The model under review builds one solid part; all positions refer to its coordinate system, in mm. Face numbers are marked on the shaded views. A direction names the side the tool comes from. Round coordinates to 2 decimals unless told otherwise and drop trailing zeros. Write each loop counter-clockwise with the first axis right and the second up, starting at its lowest first coordinate (ties: lowest second). Pieces come first, ordered by that corner, then holes. Notation, with made-up numbers: (45.5, -32.5) -> (93.5, -32.5) arc R16 ccw to (93.5, -24.5) -> close; hole circle Ø10 at (57.5, -13). An arc over 180 degrees is marked (long way). Return JSON: item names as keys, results as strings. Group by question number.
1. Take a section at B-B, the plane x = 4.75. Write out the cut boundary in (y, z), then the cut area to 3 significant figures.
2. Tool access review of the marked faces 1 and 2: name each direction out of +Z, -Z, +X, -X, +Y, -Y from which nothing blocks a thin tool from reaching the whole face with its end or side.
3. Clearance check with flat-ended pins moving along their axes: P1, Ø2, axis at y = 178.55, z = -10.5, coming from the -X side; P2, Ø0.6, axis at x = 1, y = 88.5, coming from the -Z side; P3, Ø5.5, axis at x = 11, y = 3.5, coming from the +Z side; P4, Ø5.5, axis at y = 125.12, z = -10.5, coming from the +X side. State where each tip first meets the part, or that it passes through.
4. For line 1 along Y through (x, z) = (1.2, -19); line 2 along X through (y, z) = (195, -1.65); line 3 along Z through (x, y) = (1.5, 151), list the stretches that pass through material, from the lowest coordinate up. Write a range as from..to.
5. Take a section at A-A, the plane y = 58.5. Write out the cut boundary in (x, z).
from build123d import *

# Parameters (mm, degrees)
BOSS_EXTRUDE1_DEPTH                             = 211
CSK_FOR_M3_FLAT_HEAD_MACHINE_SCREW1_D           = 3.4
CSK_FOR_M3_FLAT_HEAD_MACHINE_SCREW1_CSINK_D     = 6.3
CSK_FOR_M3_FLAT_HEAD_MACHINE_SCREW1_CSINK_ANGLE = 90
SKETCH6_W                                       = 7
SKETCH6_H                                       = 10
CUT_EXTRUDE1_DEPTH                              = 213.063669684
SKETCH7_W                                       = 7
SKETCH7_H                                       = 2.5
CUT_EXTRUDE2_DEPTH                              = 213.063669684
CSK_FOR_M3_FLAT_HEAD_MACHINE_SCREW2_D           = 3.4
CSK_FOR_M3_FLAT_HEAD_MACHINE_SCREW2_CSINK_D     = 6.3
CSK_FOR_M3_FLAT_HEAD_MACHINE_SCREW2_CSINK_ANGLE = 90
CSK_FOR_M3_FLAT_HEAD_MACHINE_SCREW3_D           = 3.4
CSK_FOR_M3_FLAT_HEAD_MACHINE_SCREW3_CSINK_D     = 6.3
CSK_FOR_M3_FLAT_HEAD_MACHINE_SCREW3_CSINK_ANGLE = 90
FILLET1_R                                       = 0.5
FILLET2_R                                       = 1
CUT_EXTRUDE3_START                              = -10
SKETCH16_R                                      = 1.7
CUT_EXTRUDE3_DEPTH                              = 10
CUT_EXTRUDE4_START                              = -10
SKETCH17_R                                      = 1.7
CUT_EXTRUDE4_DEPTH                              = 10
SKETCH20_W                                      = 2
SKETCH20_H                                      = 7.5
BOSS_EXTRUDE2_DEPTH                             = 8
SKETCH21_R                                      = 1.7
CUT_EXTRUDE5_DEPTH                              = 3


with BuildPart() as part:
    # Sketch1 → Boss-Extrude1 (new body)
    with BuildSketch(Plane(origin=(0, 0, 0), x_dir=(1, 0, 0), z_dir=(0, 1, 0))):
        Polygon((0, 15), (0, 0), (15, 0), (15, 2), (2, 2), (2, 15), align=None)
    extrude(amount=BOSS_EXTRUDE1_DEPTH)

    # CSK for M3 Flat Head Machine Screw1 (through all)
    with Locations(Plane.ZY):
        with Locations((-10.5, 178.5483), (-10.5, 150.81169946), (-10.5, 125.12070188), (-10.5, 91.71900188), (-10.5, 32.45070188), (-10.5, 79.86070188), (-10.5, 137.8117)):
            CounterSinkHole(CSK_FOR_M3_FLAT_HEAD_MACHINE_SCREW1_D / 2, CSK_FOR_M3_FLAT_HEAD_MACHINE_SCREW1_CSINK_D / 2, counter_sink_angle=CSK_FOR_M3_FLAT_HEAD_MACHINE_SCREW1_CSINK_ANGLE)

    # Sketch6 → Cut-Extrude1 (cut, through all)
    with BuildSketch(Plane.XY):
        with Locations((11.5, 206)):
            Rectangle(SKETCH6_W, SKETCH6_H)
    extrude(amount=-CUT_EXTRUDE1_DEPTH, mode=Mode.SUBTRACT)

    # Sketch7 → Cut-Extrude2 (cut, through all)
    with BuildSketch(Plane.ZY):
        with Locations((-11.5, 202.25)):
            Rectangle(SKETCH7_W, SKETCH7_H)
    extrude(amount=-CUT_EXTRUDE2_DEPTH, mode=Mode.SUBTRACT)

    # CSK for M3 Flat Head Machine Screw2 (through all)
    with Locations(Plane.ZY):
        with Locations((-11, 207.5)):
            CounterSinkHole(CSK_FOR_M3_FLAT_HEAD_MACHINE_SCREW2_D / 2, CSK_FOR_M3_FLAT_HEAD_MACHINE_SCREW2_CSINK_D / 2, counter_sink_angle=CSK_FOR_M3_FLAT_HEAD_MACHINE_SCREW2_CSINK_ANGLE)

    # CSK for M3 Flat Head Machine Screw3 (through all)
    with Locations(Plane.XY):
        with Locations((11, 3.5), (10.5, 195)):
            CounterSinkHole(CSK_FOR_M3_FLAT_HEAD_MACHINE_SCREW3_D / 2, CSK_FOR_M3_FLAT_HEAD_MACHINE_SCREW3_CSINK_D / 2, counter_sink_angle=CSK_FOR_M3_FLAT_HEAD_MACHINE_SCREW3_CSINK_ANGLE)

    # Fillet1
    fillet1_edges = [part.edges().sort_by_distance(p)[0] for p in [
        (0, 105.5, 0),
    ]]
    fillet(fillet1_edges, radius=FILLET1_R)

    # Fillet2
    fillet2_edges = [part.edges().sort_by_distance(p)[0] for p in [
        (2, 105.5, -2),
        (8, 201, -1),
        (1, 203.5, -8),
        (1, 201, -8),
    ]]
    fillet(fillet2_edges, radius=FILLET2_R)

    # Sketch16 → Cut-Extrude3 (cut)
    with BuildSketch(Plane.ZY.offset(CUT_EXTRUDE3_START)):
        with Locations((-10.5, 186.68)):
            Circle(SKETCH16_R)
        with Locations((-10.5, 111.59)):
            Circle(SKETCH16_R)
        with Locations((-10.5, 3)):
            Circle(SKETCH16_R)
        with Locations((-10.5, 178.5483)):
            Circle(SKETCH16_R)
    extrude(amount=CUT_EXTRUDE3_DEPTH, mode=Mode.SUBTRACT)

    # Sketch17 → Cut-Extrude4 (cut)
    with BuildSketch(Plane.XY.offset(CUT_EXTRUDE4_START)):
        with Locations((10.5, 186.68)):
            Circle(SKETCH17_R)
        with Locations((10.5, 111.59)):
            Circle(SKETCH17_R)
        with Locations((10.5, 10)):
            Circle(SKETCH17_R)
        with Locations((10.5, 195)):
            Circle(SKETCH17_R)
    extrude(amount=CUT_EXTRUDE4_DEPTH, mode=Mode.SUBTRACT)

    # Sketch20 → Boss-Extrude2 (add)
    with BuildSketch(Plane(origin=(0, 0, -15), x_dir=(-1, 0, 0), z_dir=(0, 0, -1))):
        with Locations((-1, 207.25)):
            Rectangle(SKETCH20_W, SKETCH20_H)
    extrude(amount=BOSS_EXTRUDE2_DEPTH)

    # Sketch21 → Cut-Extrude5 (cut)
    with BuildSketch(Plane(origin=(2, 0, 0), x_dir=(0, 0, -1), z_dir=(1, 0, 0))):
        with Locations((19, 207.5)):
            Circle(SKETCH21_R)
    extrude(amount=-CUT_EXTRUDE5_DEPTH, mode=Mode.SUBTRACT)


solid = part.part
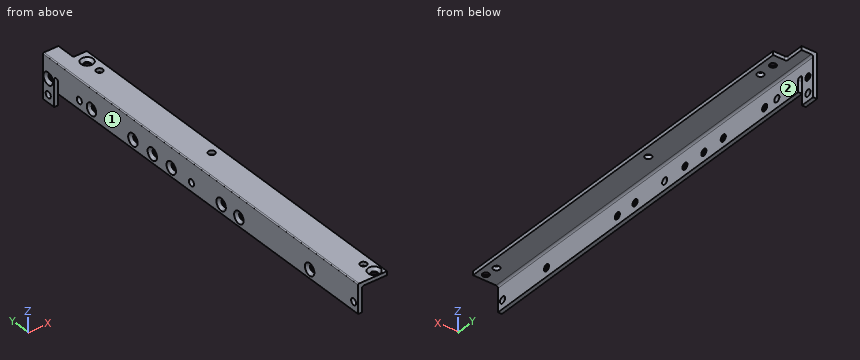
Output:
{
 "1": {"outline": "(0, -2) -> (211, -2) -> (211, 0) -> (0, 0) -> close", "area": "422 mm^2"},
 "2": {"face 1": "+Z, -Z, -X, +Y, -Y", "face 2": "-Z, +X, +Y, -Y"},
 "3": {"P1": "passes through", "P2": "stops at z = -15", "P3": "stops at z = -0.4", "P4": "stops at x = 2"},
 "4": {"line 1": "y = 203.5..205.8, 209.2..211", "line 2": "x = 0..8.8, 12.2..15", "line 3": "z = -15..-12.19, -8.81..0"},
 "5": {"outline": "(0, -15) -> (2, -15) -> (2, -3) arc R1 cw to (3, -2) -> (15, -2) -> (15, 0) -> (0.5, 0) arc R0.5 ccw to (0, -0.5) -> close"}
}
